from build123d import *

# Parameters (mm, degrees)
SKETCH1_R           = 10.922
SKETCH1_R_2         = 8.382
BOSS_EXTRUDE1_DEPTH = 9.61771
SKETCH1_3_R         = 8.382
SKETCH1_3_R_2       = 5.08
BOSS_EXTRUDE2_DEPTH = 6.60146
CHAMFER1_SIZE       = 0.762


with BuildPart() as part:
    # Sketch1 → Boss-Extrude1 (new, symmetric)
    with BuildSketch(Plane.XY):
        Circle(SKETCH1_R)
        Circle(SKETCH1_R_2, mode=Mode.SUBTRACT)
    extrude(amount=BOSS_EXTRUDE1_DEPTH, both=True)

    # Sketch1_3 → Boss-Extrude2 (add, symmetric)
    with BuildSketch(Plane.XY):
        Circle(SKETCH1_3_R)
        with Locations(Location((0, 0, 0), (0, 0, 180))):
            Circle(SKETCH1_3_R_2, mode=Mode.SUBTRACT)
    extrude(amount=BOSS_EXTRUDE2_DEPTH, both=True)

    # Chamfer1
    chamfer1_edges = [part.edges().sort_by_distance(p)[0] for p in [
        (-8.382, 0, -6.60146),
        (-8.382, 0, 6.60146),
    ]]
    chamfer(chamfer1_edges, length=CHAMFER1_SIZE)


solid = part.part
Work out the finished part from the listing and answer in its coordinate system (mm). A direction names the side the tool comes from. Coordinates: 2 decimals unless noted, no trailing zeros. Write each loop counter-clockwise with the first axis right and the second up, starting at its lowest first coordinate (ties: lowest second). Pieces come first, ordered by that corner, then holes.
1. Flat-ended cylindrical pins translate along their axes: pin 1 (6 mm diameter, centred on x = 2, y = 1, fed in from +Z); pin 2 (3 mm diameter, centred on x = -5.5, z = -6, fed in from -Y); pin 3 (10 mm diameter, centred on x = 8, z = -7, fed in from -Y); pin 4 (10 mm diameter, centred on y = -3.5, z = -1.5, fed in from -X). Find the tip coordinate at first contact, or state that the pin passes through.
Results list:
pin 1: stops at z = 6.6
pin 2: stops at y = -10.16
pin 3: stops at y = -10.5
pin 4: stops at x = -10.92
2. For a pull along X with two mould halves and no side action, classify faces 1 (the cylindrical face through (10.418, 3.281, 0.135)), 2 (the flat face through (3, -8, 9.618)), 3 (the cylindrical face through (0.661, -5.037, -0.092)), 4 (the cylindrical face through (8, 2.5, -8.5)) as +X half, -X half, draft (parallel to the pull), parting line (faces both ways), or undercut.
Results list:
face 1: parting line
face 2: draft
face 3: undercut
face 4: undercut
3. For faces 5 (the flat face through (3, -8, -9.618)), 6 (the flat face through (5, -2, -6.601)), 7 (the flat face through (5, -2, 6.601)), determine the directions among +Z, -Z, +X, -X, +Y, -Y from which every point of the face is accessible in a straight line to the end or side of a thin tool.
Results list:
face 5: -Z, +X, -X, +Y, -Y
face 6: -Z
face 7: +Z
4. The part is cut by section A-A, the plane x = 0. Write down the section's boundary in (y, z), and give its area (3 significant figures).
Results list:
outline: (-10.92, -9.62) - (-8.38, -9.62) - (-8.38, -7.36) - (-7.62, -6.6) - (-5.08, -6.6) - (-5.08, 6.6) - (-7.62, 6.6) - (-8.38, 7.36) - (-8.38, 9.62) - (-10.92, 9.62) - close; (5.08, -6.6) - (7.62, -6.6) - (8.38, -7.36) - (8.38, -9.62) - (10.92, -9.62) - (10.92, 9.62) - (8.38, 9.62) - (8.38, 7.36) - (7.62, 6.6) - (5.08, 6.6) - close
area: 186 mm2
5. The part is cut by section C-C, the plane z = 8.25. Write down the section's boundary in (x, y), and give its area (3 significant figures).
Results list:
outline: circle Ø21.84 at (0, 0); hole circle Ø16.76 at (0, 0)
area: 154 mm2
6. The part is cut by section D-D, the plane z = -5.5. Write down the section's boundary in (x, y).
Results list:
outline: circle Ø21.84 at (0, 0); hole circle Ø10.16 at (0, 0)
7. Consider line 1 along Y through (x, z) = (0, -2.25); line 2 along Y through (x, z) = (0, 8.5); line 3 along Y through (x, z) = (7, -3.75). Determine where each line is inside the solid, lowest interval first.
Results list:
line 1: y = -10.92 to -5.08, 5.08 to 10.92
line 2: y = -10.92 to -8.38, 8.38 to 10.92
line 3: y = -8.38 to 8.38
